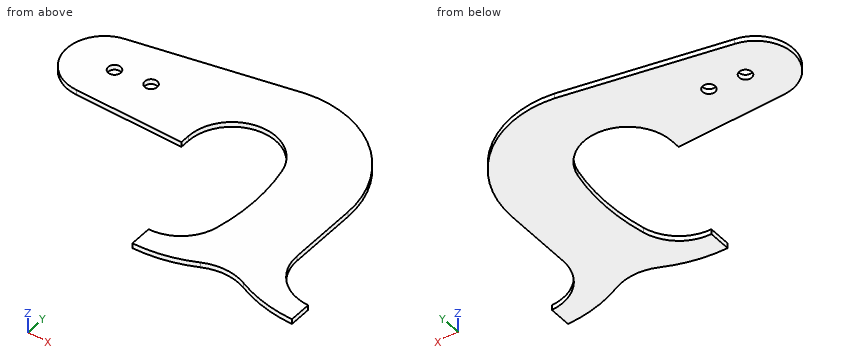
```python
from build123d import *

# Parameters (mm, degrees)
SKETCH1_R           = 12.5
BOSS_EXTRUDE1_DEPTH = 10


with BuildPart() as part:
    # Sketch1 → Boss-Extrude1 (new body)
    with BuildSketch(Plane.XY):
        with BuildLine():
            Line((231.25, 0), (231.25, -137.5))
            ThreePointArc((231.25, -137.5), (256.878155637, -199.371842345), (318.749997146, -225))
            Line((318.749997146, -225), (318.749997146, -268.75))
            ThreePointArc((318.749997146, -268.75), (259.191745399, -262.067504946), (202.595337169, -242.352341572))
            ThreePointArc((202.595337169, -242.352341572), (159.374998573, -232.529957041), (116.154659977, -242.352341572))
            ThreePointArc((116.154659977, -242.352341572), (59.558251747, -262.067504946), (0, -268.75))
            Line((0, -268.75), (0, -225))
            ThreePointArc((0, -225), (54.643732486, -205.839684664), (85.356238788, -156.75))
            ThreePointArc((85.356238788, -156.75), (95.156290044, -68.75), (85.356238788, 19.25))
            ThreePointArc((85.356238788, 19.25), (-9.68450066, 86.96240824), (-87.5, 0))
            Line((-87.5, 0), (-87.5, -18.75))
            Line((-87.5, -18.75), (-300, -14.072527462))
            ThreePointArc((-300, -14.072527462), (-374.703614676, 54.266394967), (-313.269508591, 134.744273754))
            Line((-313.269508591, 134.744273754), (0, 197.543507866))
            ThreePointArc((0, 197.543507866), (161.153810568, 152.069063257), (231.25, 0))
        make_face()
        with Locations((-281.324943498, 62.602215693)):
            Circle(SKETCH1_R, mode=Mode.SUBTRACT)
        with Locations((-212.849736322, 68.742940594)):
            Circle(SKETCH1_R, mode=Mode.SUBTRACT)
    extrude(amount=BOSS_EXTRUDE1_DEPTH)


solid = part.part
```
The listing builds one solid part. Answer for the finished solid, in the listing's coordinates (mm). Give positions to 0.01 mm unless a question says otherwise; leave off trailing zeros. Loops run counter-clockwise (first coordinate to the right, second up) from the corner with the lowest first, then second, coordinate; pieces in that order, holes last. Notation, with made-up numbers: (69, -24) - (124, -24) arc R18 cw to (124, -1) - close; hole circle Ø1 at (-2, -4.75). An arc over 180 degrees is marked (long way). Return JSON: item names as keys, results as strings. Group by question number.
1. Find section B-B (y = 26). Write down the section's boundary in (x, z), then the cut area to 3 significant figures.
2. Find section C-C (x = 163). Write down the section's boundary in (y, z), then the cut area to 3 significant figures.
3. Given pin 1 Ø5 at (y, z) = (-101, 2) entering from +X; pin 2 Ø1.5 at (x, z) = (-9.5, 5) entering from -Y; pin 3 Ø5 at (y, z) = (-256, 6) entering from -X, each flat-ended and moving along its own axis, determine where each tip first touches the part or whether it passes through.
4. Find section A-A (z = 8.5). State how many separate pieces and enclosed holes the cut face has, then the cut area to 3 significant figures.
5. Straight lines are drawn through the part: line 1 (X direction, y = 78, z = 7); line 2 (X direction, y = -69, z = 2); line 3 (X direction, y = 15.5, z = 1.25). For each, find the intervals that lie inside material, in ascending order. Write a range as [from, to].
6. Find section D-D (y = -35.5). Write down the section's boundary in (x, z), then the cut area to 3 significant figures.
Verdict:
{
 "1": {"outline": "(-366.37, 0) - (-83.55, 0) - (-83.55, 10) - (-366.37, 10) - close; (83.55, 0) - (229.55, 0) - (229.55, 10) - (83.55, 10) - close", "area": "4,290 mm^2"},
 "2": {"outline": "(-232.6, 0) - (150.47, 0) - (150.47, 10) - (-232.6, 10) - close", "area": "3,830 mm^2"},
 "3": {"pin 1": "stops at x = 231.25", "pin 2": "stops at y = 86.9", "pin 3": "stops at x = 0"},
 "4": {"separate pieces": "1", "enclosed holes": "2", "area": "131,000 mm^2"},
 "5": {"line 1": "x = [-373.03, -221.25], [-204.45, -39.65], [39.65, 215.41]", "line 2": "x = [95.16, 231.25]", "line 3": "x = [-359.68, -86.12], [86.18, 230.65]"},
 "6": {"outline": "(93.77, 0) - (231.25, 0) - (231.25, 10) - (93.77, 10) - close", "area": "1,370 mm^2"}
}
